Build history of the part. All positions in model axes, mm. Face numbers are marked on the shaded views. A direction names the side the tool comes from. Give positions to 0.01 mm unless a question says otherwise; leave off trailing zeros. Write each loop counter-clockwise with the first axis right and the second up, starting at its lowest first coordinate (ties: lowest second). Pieces come first, ordered by that corner, then holes. Notation, with made-up numbers: M 73.5,-3 L 96.5,-3 A13 ccw 96.5,18 Z; hole C 59,87.25 d11. An arc over 180 degrees is marked long. Return JSON: item names as keys, results as strings. Group by question number.
Q1. Wall check: probe 1 along Z at (x, y) = (1.25, 14.5); probe 2 along X at (y, z) = (2.5, -7.5); probe 3 along Y at (x, z) = (11, -3.5). Give the ranges that are in metal, low to high.
Q2. Tool access for the marked faces 1, 2, 3, 4 and 5: list every direction of +Z, -Z, +X, -X, +Y, -Y with a clear straight run to the whole face (end or side of a thin tool).
Q3. Band-saw the part on B-B, the plane z = 2.75. Give the cut face in (x, y).
Q4. Band-saw the part on A-A, the plane x = -3.75. Give the cut face in (y, z), then the cut area to 4 significant figures.
Q5. Flat gauge pins, fed straight in: pin 1 Ø2.5 at (x, y) = (-2.5, 10.5) entering from +Z; pin 2 Ø4 at (x, z) = (7, -9) entering from +Y; pin 3 Ø6 at (x, y) = (3, 12) entering from -Z. Where does each tip first touch, or does it go through?
Q6. Band-saw the part on C-C, the plane y = 13.25. Give the cut face in (x, z).
Q7. Band-saw the part on D-D, the plane z = -7.25. Give the cut face in (x, y).
from build123d import *

# Parameters (mm, degrees)
EXTRUDE_3_DEPTH = 15
EXTRUDE_4_DEPTH = 4
SKETCH_8_R      = 1.1
EXTRUDE_5_DEPTH = 4


with BuildPart() as part:
    # Sketch 3 → Extrude 3 (new body)
    with BuildSketch(Plane(origin=(0, 0, 0), x_dir=(1, 0, 0), z_dir=(0, 1, 0))):
        with BuildLine():
            Line((1.616451797, 11.860683611), (-6.383548203, 11.860683611))
            Line((-6.383548203, 11.860683611), (-6.383548203, 9.575683611))
            Line((-6.383548203, 9.575683611), (1.331451797, 9.575683611))
            Line((1.331451797, 9.575683611), (1.331451797, -0.924316389))
            Line((1.331451797, -0.924316389), (-6.383548203, -0.924316389))
            Line((-6.383548203, -0.924316389), (-6.383548203, -3.209316389))
            Line((-6.383548203, -3.209316389), (1.616451797, -3.209316389))
            ThreePointArc((1.616451797, -3.209316389), (3.030665359, -2.623529952), (3.616451797, -1.209316389))
            Line((3.616451797, -1.209316389), (3.616451797, 9.860683611))
            ThreePointArc((3.616451797, 9.860683611), (3.030665359, 11.274897173), (1.616451797, 11.860683611))
        make_face()
    extrude(amount=EXTRUDE_3_DEPTH)

    # Sketch 3_4 → Extrude 4 (add)
    with BuildSketch(Plane(origin=(0, 0, 0), x_dir=(1, 0, 0), z_dir=(0, 1, 0))):
        Polygon((3.616451797, 14.325683611), (3.616451797, 9.860683611), (3.616451797, -1.209316389), (3.616451797, -5.674316389), (19.616451797, -5.674316389), (19.616451797, 14.325683611), align=None)
    extrude(amount=EXTRUDE_4_DEPTH)

    # Sketch 8 → Extrude 5 (add)
    with BuildSketch(Plane(origin=(0, 4, 0), x_dir=(1, 0, 0), z_dir=(0, 1, 0))):
        with Locations(Location((7.316451797, 7.325683611, 0), (0, 0, 270))):
            Circle(SKETCH_8_R)
        with Locations(Location((15.916451797, 7.325683611, 0), (0, 0, 270))):
            Circle(SKETCH_8_R)
    extrude(amount=EXTRUDE_5_DEPTH)


solid = part.part
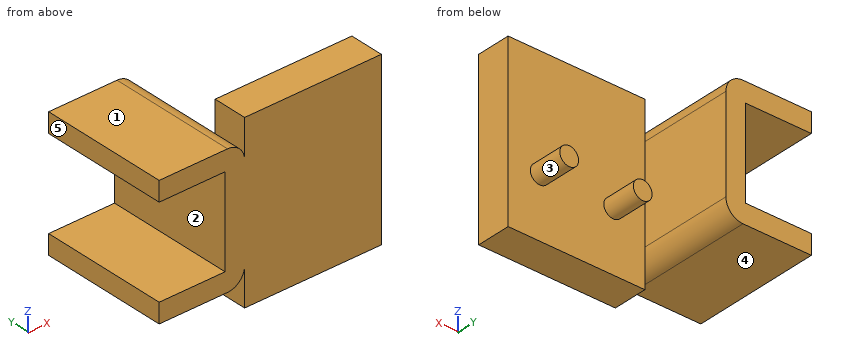
From the geometry:
{
 "1": {"probe 1": "z = -11.86 to -9.58, 0.92 to 3.21", "probe 2": "x = 1.33 to 19.62", "probe 3": "y = 0 to 4"},
 "2": {"face 1": "+Z, -X, +Y, -Y", "face 2": "-X, +Y, -Y", "face 3": "+Y", "face 4": "-Z, -X, +Y, -Y", "face 5": "+Z, -Z, -X, +Y, -Y"},
 "3": {"outline": "M -6.38,0 L 2.89,0 L 2.89,15 L -6.38,15 Z; M 3.62,0 L 19.62,0 L 19.62,4 L 3.62,4 Z"},
 "4": {"outline": "M 0,-11.86 L 15,-11.86 L 15,-9.58 L 0,-9.58 Z; M 0,0.92 L 15,0.92 L 15,3.21 L 0,3.21 Z", "area": "68.55 mm^2"},
 "5": {"pin 1": "stops at z = 3.21", "pin 2": "stops at y = 8", "pin 3": "stops at z = -11.86"},
 "6": {"outline": "M -6.38,-11.86 L 1.62,-11.86 A2 ccw 3.62,-9.86 L 3.62,1.21 A2 ccw 1.62,3.21 L -6.38,3.21 L -6.38,0.92 L 1.33,0.92 L 1.33,-9.58 L -6.38,-9.58 Z"},
 "7": {"outline": "M 1.33,0 L 19.62,0 L 19.62,4 L 17.01,4 L 17.01,8 L 14.82,8 L 14.82,4 L 8.41,4 L 8.41,8 L 6.22,8 L 6.22,4 L 3.62,4 L 3.62,15 L 1.33,15 Z"}
}
